Here's how the part is built. I have some questions about the finished solid (model axes, mm). A direction names the side the tool comes from. Coordinates: 2 decimals unless noted, no trailing zeros. Write each loop counter-clockwise with the first axis right and the second up, starting at its lowest first coordinate (ties: lowest second). Pieces come first, ordered by that corner, then holes. Notation, with made-up numbers: (56.25, 64.25) -> (113.25, 64.25) arc R33 ccw to (113.25, 101.25) -> close; hole circle Ø8 at (-14.5, 35.25). An arc over 180 degrees is marked (long way). Put each result on its own line as item: value. Start each with the question number.
Item 1: I want a section at D-D, the plane y = 16.5. List the corners of the cut face in (x, z) for me, then the cut area to 3 significant figures.
Item 2: I want a section at C-C, the plane x = -9.5. List the corners of the cut face in (y, z) for me.
Item 3: On a 3-axis mill with a long thin cutter (end or side, diameter ignored), from which of +Z, -Z, +X, -X, +Y, -Y can I reach the whole of each face in a straight line? I mean faces 5 (the face through (14.4, -2, -2)), 6 (the face through (-7, -13.1, 0)), 7 (the face through (0, 0, -3.85)). Say none if no direction works.
Item 4: I want a section at A-A, the plane y = 0. State how many separate pieces and enclosed holes the cut face has, then the cut area to 3 significant figures.
Item 5: I need wall thicknesses on line 1 (X direction, y = 15.5, z = -9.5); line 2 (Z direction, x = -15.2, y = 0); line 3 (Z direction, x = 9, y = -14). Which ranges of each line are inside material? Lowest first, please. Write a range as [from, to].
Item 6: If we mould it in two halves opening along X, with no side actions, what happens to faces 1 (the face through (15.4, 0, -16)), 2 (the face through (-7, 15, -2.4)), 3 (the face through (-13, 0, 6.25)), 4 (the face through (-15.4, 0, -11))? For each: released by +X, released by -X, zero draft, split by the parting line, or undercut.
Item 7: For pin 1 (1.4 mm diameter, centred on x = -0.5, y = 1.5, fed in from +Z); pin 2 (3 mm diameter, centred on x = 7, y = -13.5, fed in from +Z); pin 3 (2.5 mm diameter, centred on x = 4.5, y = 1, fed in from +Z); pin 4 (13 mm diameter, centred on x = -9, y = 1.5, fed in from -Z), each with a flat end and sliding along its axis, tell me the tip position at first contact or that it passes through.
from build123d import *

# Parameters (mm, degrees)
BOSS_EXTRU_1_DEPTH                                = 20
CHAMBRAGE_POUR_VIS_SIX_PANS_CREUX_M41_D           = 4.5
CHAMBRAGE_POUR_VIS_SIX_PANS_CREUX_M41_DEPTH       = 11.55
CHAMBRAGE_POUR_VIS_SIX_PANS_CREUX_M41_CBORE_D     = 8
CHAMBRAGE_POUR_VIS_SIX_PANS_CREUX_M41_CBORE_DEPTH = 1
ESQUISSE6_W                                       = 20.2
ESQUISSE6_H                                       = 20
ENL_V_MAT_EXTRU_1_DEPTH                           = 3
ESQUISSE14_W                                      = 30.8
ESQUISSE14_H                                      = 2.5
BOSS_EXTRU_3_DEPTH                                = 40
CHANFREIN1_SIZE                                   = 6.25
ESQUISSE15_W                                      = 30.8
ESQUISSE15_H                                      = 40
BOSS_EXTRU_4_DEPTH                                = 20
ENL_V_MAT_EXTRU_2_DEPTH                           = 12


with BuildPart() as part:
    # Base → Boss.-Extru.1 (new, symmetric)
    with BuildSketch(Plane(origin=(0, 0, 0), x_dir=(1, 0, 0), z_dir=(0, 1, 0))):
        Polygon((-3.85, -2.4), (-3.85, 2.4), (-10.1, 2.4), (-10.1, 10.1), (-2.4, 10.1), (-2.4, 3.85), (2.4, 3.85), (2.4, 10.1), (10.1, 10.1), (10.1, 2.4), (3.85, 2.4), (3.85, -2.4), (10.1, -2.4), (10.1, -6.25), (15.4, -6.25), (15.4, 15.4), (-15.4, 15.4), (-15.4, -6.25), (-10.1, -6.25), (-10.1, -2.4), align=None)
    extrude(amount=BOSS_EXTRU_1_DEPTH, both=True)

    # Chambrage pour vis à six pans creux M41
    with Locations(Plane(origin=(15.4, 0, 0), x_dir=(0, 0, -1), z_dir=(1, 0, 0))):
        with Locations((0, 0)):
            chambrage_pour_vis_six_pans_creux_m41 = CounterBoreHole(CHAMBRAGE_POUR_VIS_SIX_PANS_CREUX_M41_D / 2, CHAMBRAGE_POUR_VIS_SIX_PANS_CREUX_M41_CBORE_D / 2, CHAMBRAGE_POUR_VIS_SIX_PANS_CREUX_M41_CBORE_DEPTH, depth=CHAMBRAGE_POUR_VIS_SIX_PANS_CREUX_M41_DEPTH)

    # Symétrie1: Chambrage pour vis à six pans creux M41 across plane
    add(chambrage_pour_vis_six_pans_creux_m41.mirror(Plane(origin=(0, 0, 0), x_dir=(0, 0, 1), z_dir=(1, 0, 0))), mode=Mode.SUBTRACT)

    # Esquisse6 → Enlèv. mat.-Extru.1 (cut, symmetric)
    with BuildSketch(Plane.XY):
        Rectangle(ESQUISSE6_W, ESQUISSE6_H)
    extrude(amount=ENL_V_MAT_EXTRU_1_DEPTH, both=True, mode=Mode.SUBTRACT)

    # Esquisse14 → Boss.-Extru.3 (add)
    with BuildSketch(Plane.XZ.offset(20)):
        with Locations((0, -16.65)):
            Rectangle(ESQUISSE14_W, ESQUISSE14_H)
    extrude(amount=-BOSS_EXTRU_3_DEPTH)

    # Chanfrein1
    chanfrein1_edges = [part.edges().sort_by_distance(p)[0] for p in [
        (3.85, -10, 0),
        (-3.85, -10, 0),
    ]]
    chamfer(chanfrein1_edges, length=CHANFREIN1_SIZE - 0.0001)  # a hair under: the kernel refuses the full size

    # Esquisse15 → Boss.-Extru.4 (add)
    with BuildSketch(Plane(origin=(0, 0, -17.9), x_dir=(-1, 0, 0), z_dir=(0, 0, -1))):
        Rectangle(ESQUISSE15_W, ESQUISSE15_H)
    extrude(amount=BOSS_EXTRU_4_DEPTH)

    # Esquisse17 → Enlèv. mat.-Extru.2 (cut)
    with BuildSketch(Plane.ZY.offset(15.4)):
        Polygon((-37.9, -8), (-37.9, 8), (-17.9, 15), (-17.9, -15), align=None)
    extrude(amount=-ENL_V_MAT_EXTRU_2_DEPTH, mode=Mode.SUBTRACT)


solid = part.part
Calculated:
1. outline: (-15.4, -37.9) -> (15.4, -37.9) -> (15.4, 6.25) -> (10.1, 6.25) -> (10.1, 2.4) -> (3.85, 2.4) -> (3.85, -2.4) -> (10.1, -2.4) -> (10.1, -10.1) -> (2.4, -10.1) -> (2.4, -3.85) -> (-2.4, -3.85) -> (-2.4, -10.1) -> (-10.1, -10.1) -> (-10.1, -2.4) -> (-3.85, -2.4) -> (-3.85, 2.4) -> (-10.1, 2.4) -> (-10.1, 6.25) -> (-15.4, 6.25) -> close
1. area: 1,120 mm2
2. outline: (-20, -37.9) -> (-8, -37.9) -> (-15, -17.9) -> (15, -17.9) -> (8, -37.9) -> (20, -37.9) -> (20, -10.1) -> (-20, -10.1) -> close; (-20, -2.4) -> (-10.6, -2.4) -> (-10.6, 2.4) -> (-20, 2.4) -> close; (10, -2.4) -> (20, -2.4) -> (20, 2.4) -> (10, 2.4) -> close
3. face 5: +X
3. face 6: +Z
3. face 7: +Z, +Y, -Y
4. separate pieces: 3
4. enclosed holes: 0
4. area: 765 mm2
5. line 1: x = [-15.4, -10.1], [-2.4, 2.4], [10.1, 15.4]
5. line 2: z = [-17.9, -4], [4, 6.25]
5. line 3: z = [-37.9, -10.1], [-2.4, 2.4]
6. face 1: released by +X
6. face 2: undercut
6. face 3: zero draft
6. face 4: released by -X
7. pin 1: stops at z = -3.85
7. pin 2: stops at z = 2.4
7. pin 3: stops at z = -10.1
7. pin 4: stops at z = -37.9
